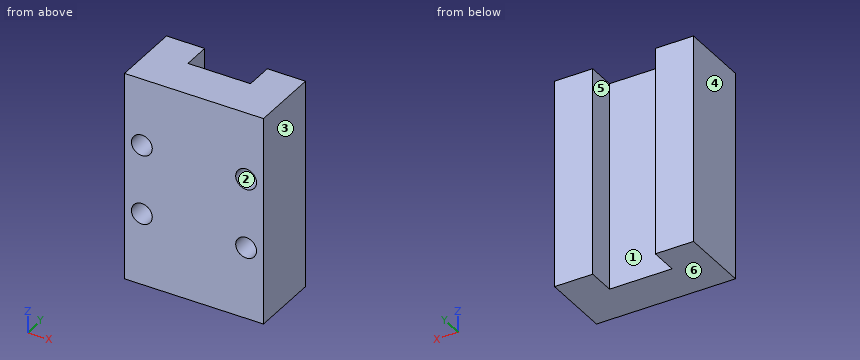
```python
from build123d import *

# Parameters (mm, degrees)
SKETCH1_W           = 20
SKETCH1_H           = 30
BOSS_EXTRUDE1_DEPTH = 10
SKETCH2_W           = 9
SKETCH2_H           = 4
CUT_EXTRUDE1_DEPTH  = 31
SKETCH3_R           = 1.5
CUT_EXTRUDE2_DEPTH  = 5


with BuildPart() as part:
    # Sketch1 → Boss-Extrude1 (new body)
    with BuildSketch(Plane(origin=(0, 0, 0), x_dir=(1, 0, 0), z_dir=(0, 1, 0))):
        with Locations((10, 15)):
            Rectangle(SKETCH1_W, SKETCH1_H)
    extrude(amount=BOSS_EXTRUDE1_DEPTH)

    # Sketch2 → Cut-Extrude1 (cut, through all)
    with BuildSketch(Plane.XY):
        with Locations((10, 8)):
            Rectangle(SKETCH2_W, SKETCH2_H)
    extrude(amount=-CUT_EXTRUDE1_DEPTH, mode=Mode.SUBTRACT)

    # Sketch3 → Cut-Extrude2 (cut)
    with BuildSketch(Plane.XZ):
        with Locations((2.5, -19.682120583)):
            Circle(SKETCH3_R)
        with Locations((17.5, -19.682120583)):
            Circle(SKETCH3_R)
        with Locations((17.5, -9.682120583)):
            Circle(SKETCH3_R)
        with Locations((2.5, -9.682120583)):
            Circle(SKETCH3_R)
    extrude(amount=-CUT_EXTRUDE2_DEPTH, mode=Mode.SUBTRACT)


solid = part.part
```
CAD build for the part. Positions are in the model's coordinates, mm. Face numbers are marked on the shaded views. A direction names the side the tool comes from. Give positions to 0.01 mm unless a question says otherwise; leave off trailing zeros. Loops run counter-clockwise (first coordinate to the right, second up) from the corner with the lowest first, then second, coordinate; pieces in that order, holes last. Notation, with made-up numbers: M 11,42 L 47,42 A31 cw 47,69 Z; hole C 9.25,87 d4. An arc over 180 degrees is marked long. Use one line per item in the form item = value.
Item 1: Slice it at A-A (y = 7.25). List the corners of the cut face in (x, z), plus the area to 3 significant figures.
Determined:
outline = M 0,-30 L 5.5,-30 L 5.5,0 L 0,0 Z; M 14.5,-30 L 20,-30 L 20,0 L 14.5,0 Z
area = 330 mm2
Item 2: Drill centre lines: probe 1 along Z at (x, y) = (2.5, 1.65); probe 2 along X at (y, z) = (6.25, -14.5); probe 3 along Y at (x, z) = (18, -8.5). Where is each one in solid material? Low to high. Write a range as from..to.
Determined:
probe_1 = -30..-21.18, -18.18..-11.18, -8.18..0
probe_2 = 0..5.5, 14.5..20
probe_3 = 5..10
Item 3: Slice it at C-C (x = 17.5). List the corners of the cut face in (y, z).
Determined:
outline = M 0,-30 L 10,-30 L 10,0 L 0,0 L 0,-8.18 L 5,-8.18 L 5,-11.18 L 0,-11.18 L 0,-18.18 L 5,-18.18 L 5,-21.18 L 0,-21.18 Z
Item 4: Two-plate mould, pull along X, no slides. Class the marked faces 4, 5 and 6: pulls with the +X half, pulls with the -X half, needs draft (parallel to the pull), parting line crosses it, or undercut.
Determined:
face_4 = pulls with the -X half
face_5 = undercut
face_6 = needs draft
Item 5: Slice it at D-D (y = 2). List the corners of the cut face in (x, z), plus the area to 3 significant figures.
Determined:
outline = M 0,-30 L 20,-30 L 20,0 L 0,0 Z; hole C 2.5,-19.68 d3; hole C 2.5,-9.68 d3; hole C 17.5,-19.68 d3; hole C 17.5,-9.68 d3
area = 572 mm2
Item 6: Flat gauge pins, fed straight in: pin 1 (2.5 mm diameter, centred on x = 17.5, z = -9.68, fed in from -Y); pin 2 (2.5 mm diameter, centred on x = 8.5, z = -19, fed in from +Y). Where does each tip first touch, or does it go through?
Determined:
pin_1 = 5
pin_2 = 6
Item 7: Slice it at B-B (z = -6.5). List the corners of the cut face in (x, y).
Determined:
outline = M 0,0 L 20,0 L 20,10 L 14.5,10 L 14.5,6 L 5.5,6 L 5.5,10 L 0,10 Z
Item 8: Which spindle directions (+Z, -Z, +X, -X, +Y, -Y) get a long thin tool onto all of the face, cutting with end or side? Do the marked faces 1, 2 and 3. Say none if no direction does.
Determined:
face_1 = +Z, -Z, +Y
face_2 = -Y
face_3 = +Z, -Z, +X, +Y, -Y
